from build123d import *

# Parameters (mm, degrees)
F0_R     = 12.5
F0_R_2   = 10.5
F0_R_3   = 1.75
F1_DEPTH = 2
F2_DEPTH = 7
F3_W     = 9
F3_H     = 1.8
F3_H_2   = 5.8387092426
F4_DEPTH = 15
F3_W_2   = 10.5
F3_H_3   = 0.2
F5_DEPTH = 6


with BuildPart() as f1:
    # F0 (on Front) → F1 (new body)
    with BuildSketch(Plane.XZ):
        Circle(F0_R)
        Circle(F0_R_2, mode=Mode.SUBTRACT)
        Circle(F0_R_2)
        Circle(F0_R_3, mode=Mode.SUBTRACT)
    extrude(amount=F1_DEPTH)

    # F0 (on Front) → F2 (join)
    with BuildSketch(Plane.XZ):
        Circle(F0_R)
        Circle(F0_R_2, mode=Mode.SUBTRACT)
    extrude(amount=-F2_DEPTH)

    # F3 (on Top) → F4 (cut, symmetric)
    with BuildSketch(Plane.XY):
        with Locations((0, 4.1)):
            Rectangle(F3_W, F3_H)
        with Locations((0, 7.9193546213)):
            Rectangle(F3_W, F3_H_2)
    extrude(amount=F4_DEPTH, both=True, mode=Mode.SUBTRACT)

    # F3 (on Top) → F5 (cut, symmetric)
    with BuildSketch(Plane.XY):
        with Locations((-9.75, 4.1)):
            Rectangle(F3_W_2, F3_H)
        with Locations((0, 7.9193546213)):
            Rectangle(F3_W, F3_H_2)
        with Locations((0, 4.1)):
            Rectangle(F3_W, F3_H)
        with Locations((9.75, 4.1)):
            Rectangle(F3_W_2, F3_H)
        with Locations((0, 3.1)):
            Rectangle(F3_W, F3_H_3)
    extrude(amount=F5_DEPTH, both=True, mode=Mode.SUBTRACT)


solid = f1.part
The model under review builds one solid part; all positions refer to its coordinate system, in mm. A direction names the side the tool comes from. Round coordinates to 2 decimals unless told otherwise and drop trailing zeros. Loops run counter-clockwise (first coordinate to the right, second up) from the corner with the lowest first, then second, coordinate; pieces in that order, holes last. Notation, with made-up numbers: (-26.75, -21) -> (11.25, -21) arc R17 cw to (11.25, -12) -> close; hole circle Ø8 at (7.25, 81). An arc over 180 degrees is marked (long way). Write item = value, one per line. Start each with the question number.
Item 1: For faces 3 (the cylindrical face through (1.617, -0.986, -0.67)), 4 (the flat face through (2, 0, 0)), 5 (the flat face through (-4.5, 5, 11)), 6 (the flat face through (10, 4, 6)), list the 3-axis set-ups (+Z, -Z, +X, -X, +Y, -Y) from which the entire face can be reached by the end or side of a thin tool; tool diameter is ignored.
Item 2: Take a section at B-B on y = 3.5. Give the boundary of the cut face in (x, z).
Item 3: Mouldability with a two-part tool opening along Z and no side actions: class faces 1 (the flat face through (4.5, 5, -11)), 2 (the flat face through (11, 3.2, 0)) as released by +Z, released by -Z, zero draft, split by the parting line, or undercut.
Item 4: Take a section at D-D on z = 0. Give the boundary of the cut face in (x, y), plus the area to 3 significant figures.
Item 5: Take a section at A-A on x = 0. Give the boundary of the cut face in (y, z).
Item 6: Insertion check: pin 1 (5 mm diameter, centred on y = 4.5, z = 2.5, fed in from -X); pin 2 (1 mm diameter, centred on x = 1.5, y = 1, fed in from +Z); pin 3 (2 mm diameter, centred on x = 10.5, y = 4.5, fed in from -Z); pin 4 (1 mm diameter, centred on x = -2, y = -0.5, fed in from -Z). Each pin has a flat end and moves straight along its axis. Give the tip position at first contact, or say it passes through.
Item 7: To check wall thickness, follow L1, parallel to Z at x = 0.25, y = 1.75; L2, parallel to Y at x = 11, z = 4.75; L3, parallel to Z at x = 0, y = -1.2. State the ranges of each line that lie inside material, in increasing order.
Item 8: Take a section at C-C on z = 2.5. Give the boundary of the cut face in (x, y).
Result:
q1.face_3 = +Y, -Y
q1.face_4 = +Y
q1.face_5 = +Z, -Z, +Y
q1.face_6 = +X, -X
q2.outline = (-10.97, -6) arc R12.5 ccw to (-4.5, -11.66) -> (-4.5, -9.49) arc R10.5 cw to (-8.62, -6) -> close; (-10.97, 6) -> (-8.62, 6) arc R10.5 cw to (-4.5, 9.49) -> (-4.5, 11.66) arc R12.5 ccw to start; (4.5, -11.66) arc R12.5 ccw to (10.97, -6) -> (8.62, -6) arc R10.5 cw to (4.5, -9.49) -> close; (4.5, 9.49) arc R10.5 cw to (8.62, 6) -> (10.97, 6) arc R12.5 ccw to (4.5, 11.66) -> close
q3.face_1 = zero draft
q3.face_2 = undercut
q4.outline = (-12.5, -2) -> (-1.75, -2) -> (-1.75, 0) -> (-10.5, 0) -> (-10.5, 3.2) -> (-12.5, 3.2) -> close; (-12.5, 5) -> (-10.5, 5) -> (-10.5, 7) -> (-12.5, 7) -> close; (1.75, -2) -> (12.5, -2) -> (12.5, 3.2) -> (10.5, 3.2) -> (10.5, 0) -> (1.75, 0) -> close; (10.5, 5) -> (12.5, 5) -> (12.5, 7) -> (10.5, 7) -> close
q4.area = 63.8 mm²
q5.outline = (-2, -12.5) -> (3.2, -12.5) -> (3.2, -10.5) -> (0, -10.5) -> (0, -1.75) -> (-2, -1.75) -> close; (-2, 1.75) -> (0, 1.75) -> (0, 10.5) -> (3.2, 10.5) -> (3.2, 12.5) -> (-2, 12.5) -> close
q6.pin_1 = -12.5
q6.pin_2 = 12.46
q6.pin_3 = -8.12
q6.pin_4 = -12.41
q7.L1 = -12.5 to -10.5, 10.5 to 12.5
q7.L2 = -2 to 3.2, 5 to 7
q7.L3 = -12.5 to -1.75, 1.75 to 12.5
q8.outline = (-12.25, -2) -> (12.25, -2) -> (12.25, 3.2) -> (10.2, 3.2) -> (10.2, 0) -> (-10.2, 0) -> (-10.2, 3.2) -> (-12.25, 3.2) -> close; (-12.25, 5) -> (-10.2, 5) -> (-10.2, 7) -> (-12.25, 7) -> close; (10.2, 5) -> (12.25, 5) -> (12.25, 7) -> (10.2, 7) -> close
